Design review of the part shown in the three views and the two pictorial views. Dimensions are in mm from the part's minimum x, y and z. A direction names the side the tool comes from. Coordinates: 2 decimals unless noted, no trailing zeros. Loops run counter-clockwise (first coordinate to the right, second up) from the corner with the lowest first, then second, coordinate; pieces in that order, holes last. Notation, with made-up numbers: (59, -17) - (94, -17) arc R19 ccw to (94, 5) - close; hole circle Ø10 at (63, -13.5). An arc over 180 degrees is marked (long way). One line per question, with ' | ' between items.
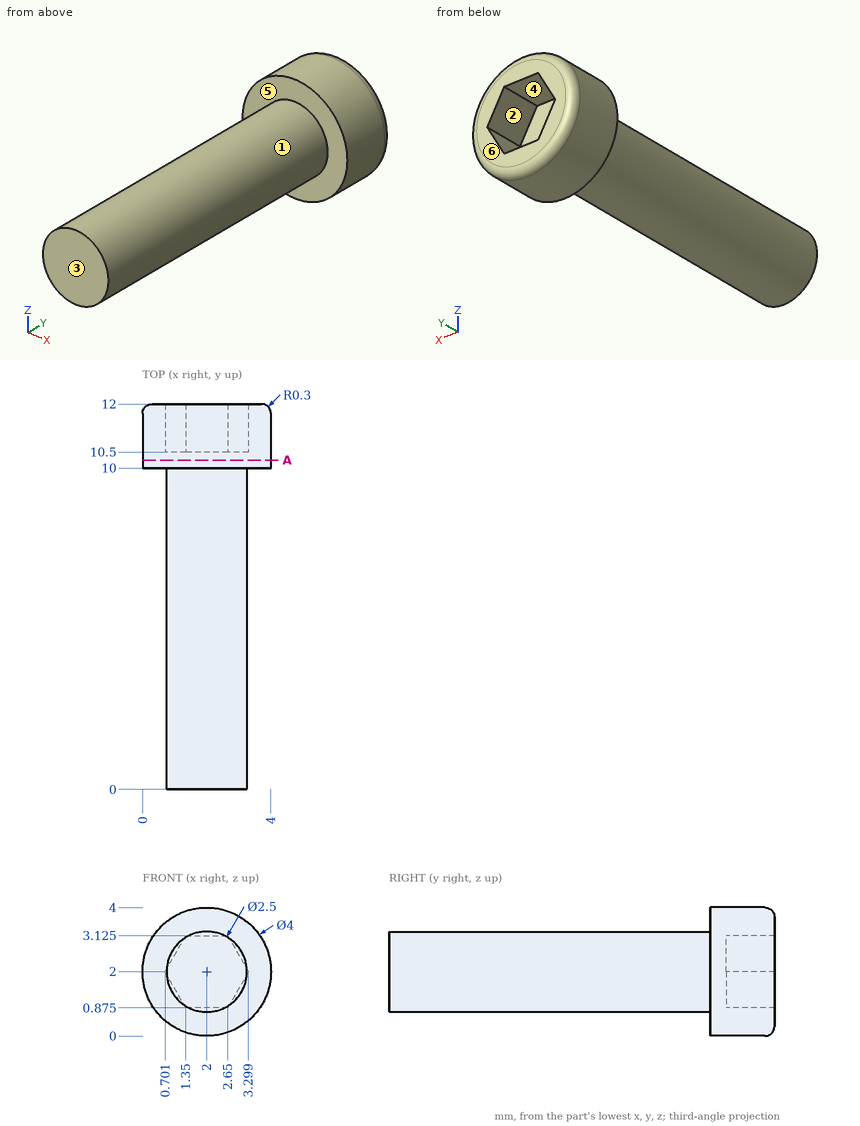
Q1. To check wall thickness, follow line 1 along Y through (x, z) = (1.8, 0.55); line 2 along Y through (x, z) = (1.2, 1.4); line 3 along X through (y, z) = (11, 2.1). State the ranges of each line that lie inside material, in increasing order.
Returned:
line 1: y = 10 to 12 | line 2: y = 0 to 10.5 | line 3: x = 0 to 0.76, 3.24 to 4
Q2. Draft analysis for pull direction Z (two halves, no side actions). For the marked faces 1, 2, 3 and 4, state which applies: +Z half, -Z half, draft (parallel to the pull), parting line (faces both ways), or undercut.
Returned:
face 1: parting line | face 2: undercut | face 3: draft | face 4: undercut
Q3. For pin 1 (0.7 mm diameter, centred on x = 1.5, z = 1.5, fed in from +Y); pin 2 (1 mm diameter, centred on x = 3.5, y = 10, fed in from -Z), all flat-tipped, find the tip position at first contact; note any pin that passes through.
Returned:
pin 1: stops at y = 10.5 | pin 2: stops at z = 0.27
Q4. Take a section at A-A (y = 10.25). Give the boundary of the cut face in (x, z), plus the area to 3 significant figures.
Returned:
outline: circle Ø4 at (2, 2) | area: 12.6 mm²
Q5. Tool access review of the marked faces 5 and 6: name each direction out of +Z, -Z, +X, -X, +Y, -Y from which nothing blocks a thin tool from reaching the whole face with its end or side.
Returned:
face 5: -Y | face 6: +Z, -Z, +X, -X, +Y
